```python
from build123d import *

# Parameters (mm, degrees)
SKETCH1_R           = 2.667
BOSS_EXTRUDE1_DEPTH = 139.7
SKETCH2_R           = 1.524
CUT_EXTRUDE1_DEPTH  = 5.08
SKETCH5_R           = 1.524
CUT_EXTRUDE2_DEPTH  = 5.08


with BuildPart() as part:
    # Sketch1 → Boss-Extrude1 (new body)
    with BuildSketch(Plane.XY):
        with BuildLine():
            ThreePointArc((0.134056593, 2.54), (0.077982482, -1.938389365), (0.85051547, -6.35))
            Line((0.85051547, -6.35), (47.40948453, -6.35))
            ThreePointArc((47.40948453, -6.35), (48.182017518, -1.938389365), (48.125943407, 2.54))
            Line((48.125943407, 2.54), (0.134056593, 2.54))
        make_face()
        with Locations((43.18, -1.634887509)):
            Circle(SKETCH1_R, mode=Mode.SUBTRACT)
        with Locations((5.08, -1.634887509)):
            Circle(SKETCH1_R, mode=Mode.SUBTRACT)
    extrude(amount=BOSS_EXTRUDE1_DEPTH)

    # Sketch2 → Cut-Extrude1 (cut)
    with BuildSketch(Plane(origin=(0, 2.54, 0), x_dir=(1, 0, 0), z_dir=(0, 1, 0))):
        with Locations((17.145, -7.62)):
            Circle(SKETCH2_R)
        with Locations((31.115, -7.62)):
            Circle(SKETCH2_R)
        with Locations((31.115, -39.37)):
            Circle(SKETCH2_R)
        with Locations((17.145, -39.37)):
            Circle(SKETCH2_R)
        with Locations((17.78, -55.88)):
            Circle(SKETCH2_R)
        with Locations((30.48, -55.88)):
            Circle(SKETCH2_R)
        with Locations((30.48, -85.09)):
            Circle(SKETCH2_R)
        with Locations((17.78, -85.09)):
            Circle(SKETCH2_R)
        with Locations((16.51, -129.54)):
            Circle(SKETCH2_R)
        with Locations((31.75, -129.54)):
            Circle(SKETCH2_R)
    extrude(amount=-CUT_EXTRUDE1_DEPTH, mode=Mode.SUBTRACT)

    # Sketch5 → Cut-Extrude2 (cut)
    with BuildSketch(Plane.XZ.offset(6.35)):
        with Locations((17.78, 125.73)):
            Circle(SKETCH5_R)
        with Locations((30.48, 125.73)):
            Circle(SKETCH5_R)
        with Locations((30.48, 100.33)):
            Circle(SKETCH5_R)
        with Locations((17.78, 100.33)):
            Circle(SKETCH5_R)
    extrude(amount=-CUT_EXTRUDE2_DEPTH, mode=Mode.SUBTRACT)


solid = part.part
```
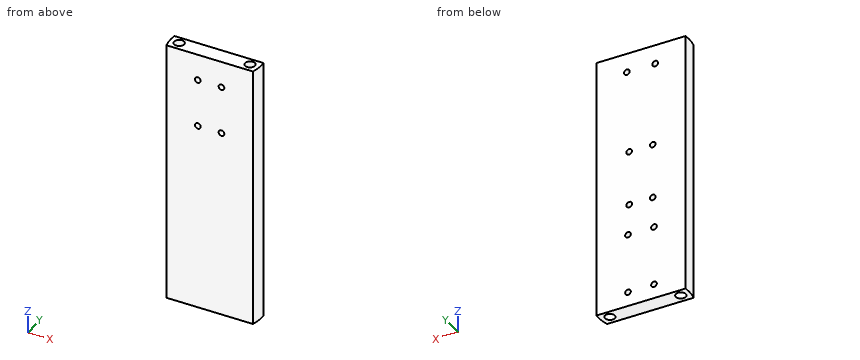
The model under review builds one solid part; all positions refer to its coordinate system, in mm. Coordinates: 2 decimals unless noted, no trailing zeros. Write each loop counter-clockwise with the first axis right and the second up, starting at its lowest first coordinate (ties: lowest second). Pieces come first, ordered by that corner, then holes. Notation, with made-up numbers: (28.5, -12) - (82.5, -12) arc R10 ccw to (82.5, 6) - close; hole circle Ø6 at (-22.75, 61.5). An arc over 180 degrees is marked (long way). Answer in a Markdown table with one row per item. Add a question column.
Q1. Consider section A-A on x = 5.08. Give the boundary of the cut face in (y, z).
Q2. Clearance check with flat-ended pins moving along their axes: pin 1 (2.5 mm diameter, centred on x = 17.78, z = 100.33, fed in from -Y); pin 2 (1.5 mm diameter, centred on x = 31.5, z = 39, fed in from +Y); pin 3 (1 mm diameter, centred on y = -1, z = 74.5, fed in from +X). State where each tip first meets the part, or that it passes through.
Q3. Consider section B-B on z = 85.09. Give the boundary of the cut face in (x, y), then the cut area to 3 significant figures.
Q4. To check wall thickness, follow line 1 along Z through (x, y) = (30.48, -4.45); line 2 along X through (y, z) = (-2.5, 34); line 3 along X through (y, z) = (0, 51). State the ranges of each line that lie inside material, in increasing order. Write a range as from..to.
Q5. Consider section D-D on z = 23.5. Give the boundary of the cut face in (x, y), then the cut area to 3 significant figures.
Answers below:
| question | item | result |
|---|---|---|
| 1 | outline | (-6.35, 0) - (-4.3, 0) - (-4.3, 139.7) - (-6.35, 139.7) - close; (1.03, 0) - (2.54, 0) - (2.54, 139.7) - (1.03, 139.7) - close |
| 2 | pin 1 | y = -1.27 |
| 2 | pin 2 | y = -2.54 |
| 2 | pin 3 | x = 48.25 |
| 3 | outline | (0.13, 2.54) arc R24.13 ccw to (0.85, -6.35) - (47.41, -6.35) arc R24.13 ccw to (48.13, 2.54) - (32, 2.54) - (32, -2.54) - (28.96, -2.54) - (28.96, 2.54) - (19.3, 2.54) - (19.3, -2.54) - (16.26, -2.54) - (16.26, 2.54) - close; hole circle Ø5.33 at (5.08, -1.63); hole circle Ø5.33 at (43.18, -1.63) |
| 3 | area | 350 mm² |
| 4 | line 1 | 0..98.81, 101.85..124.21, 127.25..139.7 |
| 4 | line 2 | 0.13..2.56, 7.6..40.66, 45.7..48.13 |
| 4 | line 3 | 0..2.97, 7.19..41.07, 45.29..48.26 |
| 5 | outline | (0.13, 2.54) arc R24.13 ccw to (0.85, -6.35) - (47.41, -6.35) arc R24.13 ccw to (48.13, 2.54) - close; hole circle Ø5.33 at (5.08, -1.63); hole circle Ø5.33 at (43.18, -1.63) |
| 5 | area | 381 mm² |
